Work out the finished part from the listing and answer in its coordinate system (mm). Round coordinates to 2 decimals unless told otherwise and drop trailing zeros. Write each loop counter-clockwise with the first axis right and the second up, starting at its lowest first coordinate (ties: lowest second). Pieces come first, ordered by that corner, then holes.
1. Flat-ended cylindrical pins translate along their axes: pin 1 Ø2.5 at (x, y) = (0, -61) entering from +Z; pin 2 Ø4 at (y, z) = (31.5, -13.5) entering from +X; pin 3 Ø3 at (x, z) = (-40.5, -11.5) entering from -Y. Find the tip coordinate at first contact, or state that the pin passes through.
2. Find section A-A (y = 0). Write down the section's boundary in (x, z).
3. Straight lines are drawn through the part: probe 1 along Y at (x, z) = (0, -7.5); probe 2 along Y at (x, z) = (0, -16.75); probe 3 along X at (y, z) = (-30.5, -7.25). For each, find the intervals that lie inside material, in ascending order.
4. Determine the mould class of faces 1 (the face through (-43.765, -33.558, -10.452)), 2 (the face through (60.967, -25.278, -10.853)), 3 (the face through (-34, 44, 0)) for opening direction X: pulls with the +X half, pulls with the -X half, needs draft (parallel to the pull), parting line crosses it, or undercut.
5. Find section B-B (z = -14.75). Write down the section's boundary in (x, y), and give its area (3 significant figures).
```python
from build123d import *

# Parameters (mm, degrees)
SKETCH1_R                       = 66
SKETCH1_R_2                     = 55.15
COLLAR_BODY_DEPTH               = 22
M4PATTERN_COUNT                 = 6
F_3_0MM_DOWEL_HOLE5_D           = 3
F_3_0MM_DOWEL_HOLE5_DEPTH       = 7
F_3_0MM_DOWEL_HOLE5_CSINK_D     = 3.05
F_3_0MM_DOWEL_HOLE5_CSINK_ANGLE = 90
F_3_0MM_DOWEL_HOLE5_TIP         = 0.901290929
CHAMFER1_SIZE                   = 0.5
CHAMFER2_SIZE                   = 0.8


with BuildPart() as part:
    # Sketch1 → Collar_Body (new body)
    with BuildSketch(Plane.XY):
        Circle(SKETCH1_R)
        Circle(SKETCH1_R_2, mode=Mode.SUBTRACT)
    extrude(amount=-COLLAR_BODY_DEPTH)

    # Sketch5 → M4x0.7 Bottoming Tapped Hole1 (revolve, cut)
    with BuildSketch(Plane(origin=(0, 61, 0), x_dir=(0, -1, 0), z_dir=(1, 0, 0))):
        Polygon((0, 0), (0, 11.991420021), (1.65, 11), (1.65, 0.375), (2.025, 0), align=None)
    m4x0_7_bottoming_tapped_hole1 = revolve(axis=Axis((0, 61, 6.35), (0, 0, -1)), mode=Mode.SUBTRACT)

    # M4pattern: M4x0.7 Bottoming Tapped Hole1 ×6 about axis
    m4pattern_axis = Axis((0, 0, 0), (0, 0, 1))
    for i in range(1, M4PATTERN_COUNT):
        add(m4x0_7_bottoming_tapped_hole1.rotate(m4pattern_axis, i * 360 / M4PATTERN_COUNT), mode=Mode.SUBTRACT)

    # Ø3.0mm Dowel Hole5
    with Locations(Plane.XY):
        with Locations((30.5, 52.827549631)):
            CounterSinkHole(F_3_0MM_DOWEL_HOLE5_D / 2, F_3_0MM_DOWEL_HOLE5_CSINK_D / 2, depth=F_3_0MM_DOWEL_HOLE5_DEPTH, counter_sink_angle=F_3_0MM_DOWEL_HOLE5_CSINK_ANGLE)
            with Locations((0, 0, -(F_3_0MM_DOWEL_HOLE5_DEPTH + F_3_0MM_DOWEL_HOLE5_TIP / 2))):  # 118° drill point
                Cone(0, F_3_0MM_DOWEL_HOLE5_D / 2, F_3_0MM_DOWEL_HOLE5_TIP, mode=Mode.SUBTRACT)

    # Chamfer1
    chamfer1_edges = [part.edges().sort_by_distance(p)[0] for p in [
        (-66, 0, 0),
        (-66, 0, -22),
    ]]
    chamfer(chamfer1_edges, length=CHAMFER1_SIZE)

    # Chamfer2
    chamfer2_edges = [part.edges().sort_by_distance(p)[0] for p in [
        (-55.15, 0, -22),
    ]]
    chamfer(chamfer2_edges, length=CHAMFER2_SIZE)


solid = part.part
```
Worked answers:
1. pin 1: stops at z = -11.24
1. pin 2: stops at x = 59.04
1. pin 3: stops at y = -53.24
2. outline: (-66, -21.5) - (-65.5, -22) - (-55.95, -22) - (-55.15, -21.2) - (-55.15, 0) - (-65.5, 0) - (-66, -0.5) - close; (55.15, -21.2) - (55.95, -22) - (65.5, -22) - (66, -21.5) - (66, -0.5) - (65.5, 0) - (55.15, 0) - close
3. probe 1: y = -66 to -62.65, -59.35 to -55.15, 55.15 to 59.35, 62.65 to 66
3. probe 2: y = -66 to -55.15, 55.15 to 66
3. probe 3: x = -58.53 to -54.48, -51.18 to -45.95, 45.95 to 51.18, 54.48 to 58.53
4. face 1: undercut
4. face 2: parting line crosses it
4. face 3: needs draft
5. outline: circle Ø132 at (0, 0); hole circle Ø110.3 at (0, 0)
5. area: 4,130 mm2
